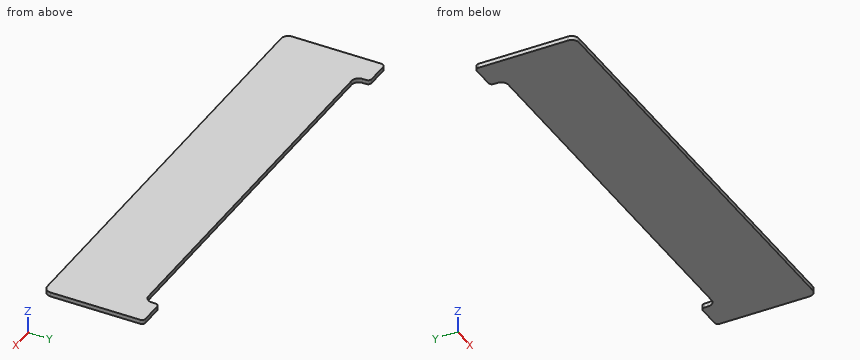
```python
from build123d import *

# Parameters (mm, degrees)
SKETCH1_W           = 315
SKETCH1_H           = 70
BOSS_EXTRUDE1_DEPTH = 3
SKETCH2_W           = 275
SKETCH2_H           = 10
CUT_EXTRUDE1_DEPTH  = 3
FILLET1_R           = 5
FILLET2_R           = 2.5


with BuildPart() as part:
    # Sketch1 → Boss-Extrude1 (new body)
    with BuildSketch(Plane.XY):
        Rectangle(SKETCH1_W, SKETCH1_H)
    extrude(amount=BOSS_EXTRUDE1_DEPTH)

    # Sketch2 → Cut-Extrude1 (cut)
    with BuildSketch(Plane.XY.offset(3)):
        with Locations((0, 30)):
            Rectangle(SKETCH2_W, SKETCH2_H)
    extrude(amount=-CUT_EXTRUDE1_DEPTH, mode=Mode.SUBTRACT)

    # Fillet1
    fillet1_edges = [part.edges().sort_by_distance(p)[0] for p in [
        (-137.5, 25, 1.5),
        (137.5, 25, 1.5),
        (157.5, -35, 1.5),
        (-157.5, -35, 1.5),
    ]]
    fillet(fillet1_edges, radius=FILLET1_R)

    # Fillet2
    fillet2_edges = [part.edges().sort_by_distance(p)[0] for p in [
        (-137.5, 35, 1.5),
        (137.5, 35, 1.5),
        (-157.5, 35, 1.5),
        (157.5, 35, 1.5),
    ]]
    fillet(fillet2_edges, radius=FILLET2_R)


solid = part.part
```
Work out the finished part from the listing and answer in its coordinate system (mm). Give positions to 0.01 mm unless a question says otherwise; leave off trailing zeros. Loops run counter-clockwise (first coordinate to the right, second up) from the corner with the lowest first, then second, coordinate; pieces in that order, holes last. Notation, with made-up numbers: (59, 17) - (65, 17) arc R19 cw to (65, 25) - close; hole circle Ø2 at (40, 70). An arc over 180 degrees is marked (long way). One line per question, with ' | ' between items.
(1) Straight lines are drawn through the part: probe 1 along X at (y, z) = (31.5, 1.9); probe 2 along Y at (x, z) = (97, 0.8); probe 3 along X at (y, z) = (27.5, 1.75). For each, find the intervals that lie inside material, in ascending order.
Recorded:
probe 1: x = -157.5 to -137.5, 137.5 to 157.5 | probe 2: y = -35 to 25 | probe 3: x = -157.5 to -136.83, 136.83 to 157.5
(2) This flat-tipped pin is pushed along its axis until it touches: pin 1 Ø1 at (x, z) = (-54.5, 1) entering from +Y. Where does it stop, or does it pass through?
Recorded:
pin 1: stops at y = 25
(3) The part is cut by section A-A (z = 2.25). Write down the section's boundary in (x, y), then the cut area to 3 significant figures.
Recorded:
outline: (-157.5, -30) arc R5 ccw to (-152.5, -35) - (152.5, -35) arc R5 ccw to (157.5, -30) - (157.5, 32.5) arc R2.5 ccw to (155, 35) - (140, 35) arc R2.5 ccw to (137.5, 32.5) - (137.5, 30) arc R5 cw to (132.5, 25) - (-132.5, 25) arc R5 cw to (-137.5, 30) - (-137.5, 32.5) arc R2.5 ccw to (-140, 35) - (-155, 35) arc R2.5 ccw to (-157.5, 32.5) - close | area: 19,300 mm²
(4) The part is cut by section B-B (x = -8). Write down the section's boundary in (y, z), then the cut area to 3 significant figures.
Recorded:
outline: (-35, 0) - (25, 0) - (25, 3) - (-35, 3) - close | area: 180 mm²
